CAD build for the part. Positions are in the model's coordinates, mm. Face numbers are marked on the shaded views. A direction names the side the tool comes from. Coordinates: 2 decimals unless noted, no trailing zeros. Write each loop counter-clockwise with the first axis right and the second up, starting at its lowest first coordinate (ties: lowest second). Pieces come first, ordered by that corner, then holes. Notation, with made-up numbers: (53, 89) - (66, 89) arc R24 cw to (66, 99) - close; hole circle Ø8 at (32.5, 59.25). An arc over 180 degrees is marked (long way). Answer in a Markdown table with one row per item. Add a question column.
Q1. 3-axis set-ups, long thin cutter, end or side, ignore diameter. For the marked faces 1, 2 and 3: which of +Z, -Z, +X, -X, +Y, -Y reach the whole face in a straight line?
Q2. Band-saw the part on A-A (y = 73.5). List the corners of the cut face in (x, z), and give its area (3 significant figures).
Q3. Drill centre lines: line 1 along Y through (x, z) = (-5.25, -3); line 2 along Y through (x, z) = (1.75, 1.5); line 3 along X through (y, z) = (17.5, -5.75). Where is each one in solid material? Low to high. Write a range as from..to.
Q4. Pin check, flat tips, straight feed: pin 1 (1.5 mm diameter, centred on x = -0.5, y = 3.5, fed in from +Z); pin 2 (1 mm diameter, centred on x = 2, z = 3.5, fed in from -Y); pin 3 (2 mm diameter, centred on x = -2.5, y = 85.5, fed in from -Z). Stop position of each tip, or through.
Q5. Two-plate mould, pull along Z, no slides. Class the marked faces 4, 5 and 6: +Z half, -Z half, draft (parallel to the pull), parting line (faces both ways), or undercut.
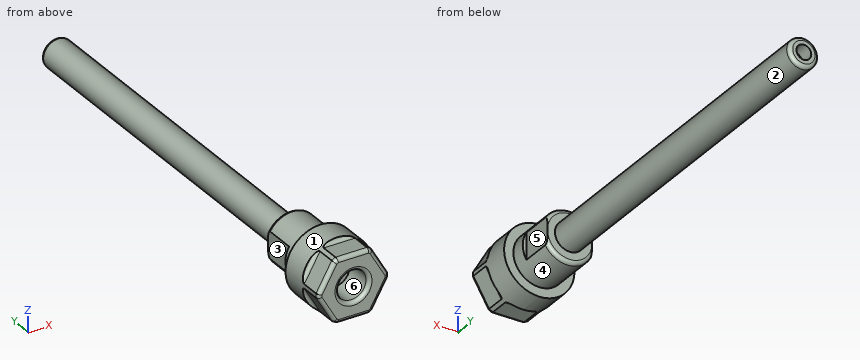
```python
from build123d import *

# Parameters (mm, degrees)
ESQUISSE2_R             = 4
ENL_V_MAT_EXTRU_1_DEPTH = 8
ENL_V_START             = -9
ENL_V_MAT_EXTRU_2_DEPTH = 9
ESQUISSE4_R             = 15
ENL_V_MAT_EXTRU_3_DEPTH = 7
CONG_1_R                = 1


with BuildPart() as part:
    # Esquisse1 → Révolution1 (revolve)
    with BuildSketch(Plane.XY, mode=Mode.PRIVATE) as r_volution1_sk:
        Polygon((4, 127), (4, 27), (7, 27), (7, 14), (9.5, 14), (9.5, 0), (0, 0), (0, 121), (2, 123), (2, 127), align=None)
    revolve(r_volution1_sk.sketch.rotate(Axis((0, 0, 0), (0, 1, 0)), 90), axis=Axis((0, 0, 0), (0, 1, 0)))

    # Esquisse2 → Enlèv. mat.-Extru.1 (cut)
    with BuildSketch(Plane.XZ):
        with Locations(Location((0, 0, 0), (0, 0, 270))):
            Circle(ESQUISSE2_R)
    extrude(amount=-ENL_V_MAT_EXTRU_1_DEPTH, mode=Mode.SUBTRACT)

    # Esquisse3 → Enlèv. mat.-Extru.2 (cut)
    with BuildSketch(Plane(origin=(0, 27, 0), x_dir=(1, 0, 0), z_dir=(0, 1, 0)).offset(ENL_V_START)):
        with BuildLine():
            Line((6, -3.605551275), (6, 3.605551275))
            ThreePointArc((6, 3.605551275), (7, 0), (6, -3.605551275))
        make_face()
        with BuildLine():
            Line((-6, -3.605551275), (-6, 3.605551275))
            ThreePointArc((-6, 3.605551275), (-7, 0), (-6, -3.605551275))
        make_face()
    extrude(amount=ENL_V_MAT_EXTRU_2_DEPTH, mode=Mode.SUBTRACT)

    # Esquisse4 → Enlèv. mat.-Extru.3 (cut)
    with BuildSketch(Plane.XZ):
        Circle(ESQUISSE4_R)
        Polygon((9.814954576, 0), (4.907477288, 8.5), (-4.907477288, 8.5), (-9.814954576, 0), (-4.907477288, -8.5), (4.907477288, -8.5), align=None, mode=Mode.SUBTRACT)
    extrude(amount=-ENL_V_MAT_EXTRU_3_DEPTH, mode=Mode.SUBTRACT)

    # Congé1
    cong_1_edges = [part.edges().sort_by_distance(p)[0] for p in [
        (0, 127, 4),
        (-3.446820352, 27, -6.092571663),
        (0, 27, 7),
        (0, 0, -8.5),
        (-4.75, 0, -8.227241336),
        (-7.361215932, 0, -4.25),
        (-9.5, 0, 0),
        (-7.361215932, 0, 4.25),
        (-4.75, 0, 8.227241336),
        (0, 0, 8.5),
        (4.75, 0, 8.227241336),
        (7.361215932, 0, 4.25),
        (9.5, 0, 0),
        (7.361215932, 0, -4.25),
        (4.75, 0, -8.227241336),
        (0, 0, 4),
        (0, 7, 8.5),
        (7.361215932, 7, 4.25),
        (7.361215932, 7, -4.25),
        (0, 7, -8.5),
        (-7.361215932, 7, -4.25),
        (-7.361215932, 7, 4.25),
    ]]
    fillet(cong_1_edges, radius=CONG_1_R - 0.0001)  # a hair under: the kernel refuses the full size


solid = part.part
```
Checked values:
| question | item | result |
|---|---|---|
| 1 | face 1 | +Y, -Y |
| 1 | face 2 | +Y |
| 1 | face 3 | +Z, -Z, -X, +Y |
| 2 | outline | circle Ø8 at (0, 0) |
| 2 | area | 50.3 mm² |
| 3 | line 1 | y = 0..27 |
| 3 | line 2 | y = 8..127 |
| 3 | line 3 | x = -3.99..3.99 |
| 4 | pin 1 | stops at z = 8.5 |
| 4 | pin 2 | stops at y = 0.12 |
| 4 | pin 3 | stops at z = -3.71 |
| 5 | face 4 | parting line |
| 5 | face 5 | draft |
| 5 | face 6 | undercut |
